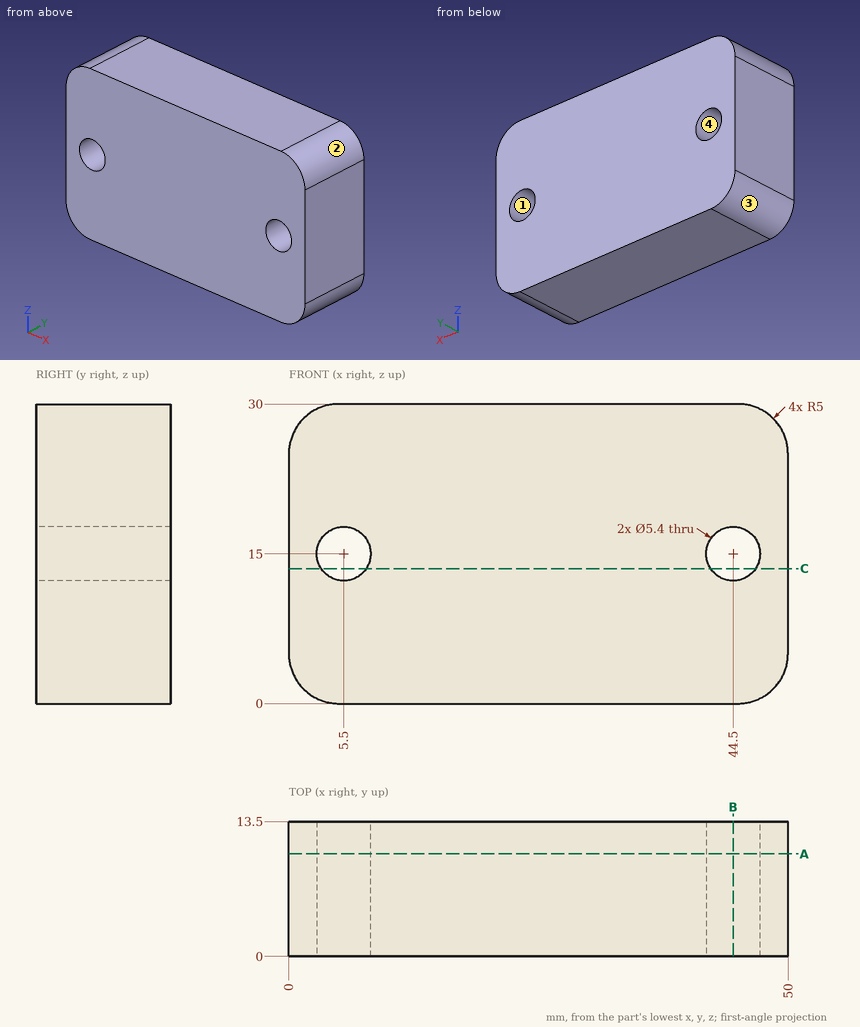
The figure shows three views and two pictorial views of one solid part (mm, origin at its lowest corner). Answer the questions. Give positions to 0.01 mm unless a question says otherwise; leave off trailing zeros. Write each loop counter-clockwise with the first axis right and the second up, starting at its lowest first coordinate (ties: lowest second). Pieces come first, ordered by that corner, then holes. Notation, with made-up numbers: M -32.75,45 L -18.75,45 A22 ccw -18.75,77 Z; hole C 41.25,59 d4. An arc over 180 degrees is marked long. Write each question's results on one line, items separated by ' | '.
Q1. Section B-B, the plane x = 44.5 is taken. Write down the section's boundary in (y, z).
Output values:
outline: M 0,0 L 13.5,0 L 13.5,12.3 L 0,12.3 Z; M 0,17.7 L 13.5,17.7 L 13.5,30 L 0,30 Z
Q2. Consider L1, parallel to X at y = 6.75, z = 15; L2, parallel to Z at x = 5.5, y = 8; L3, parallel to Z at x = 7, y = 4 (3 decimals). Determine where each line is inside the solid, lowest interval first. Write a range as from..to.
Output values:
L1: 0..2.8, 8.2..41.8, 47.2..50 | L2: 0..12.3, 17.7..30 | L3: 0..12.755, 17.245..30
Q3. Section C-C, the plane z = 13.5 is taken. Write down the section's boundary in (x, y) (3 decimals).
Output values:
outline: M 0,0 L 3.255,0 L 3.255,13.5 L 0,13.5 Z; M 7.745,0 L 42.255,0 L 42.255,13.5 L 7.745,13.5 Z; M 46.745,0 L 50,0 L 50,13.5 L 46.745,13.5 Z
Q4. For a pull along Z with two mould halves and no side action, classify the marked faces 1, 2, 3 and 4 as released by +Z, released by -Z, zero draft, split by the parting line, or undercut.
Output values:
face 1: undercut | face 2: released by +Z | face 3: released by -Z | face 4: undercut
Q5. Section A-A, the plane y = 10.25 is taken. Write down the section's boundary in (x, z).
Output values:
outline: M 0,5 A5 ccw 5,0 L 45,0 A5 ccw 50,5 L 50,25 A5 ccw 45,30 L 5,30 A5 ccw 0,25 Z; hole C 5.5,15 d5.4; hole C 44.5,15 d5.4
